The model under review builds one solid part; all positions refer to its coordinate system, in mm. A direction names the side the tool comes from. Give positions to 0.01 mm unless a question says otherwise; leave off trailing zeros. Loops run counter-clockwise (first coordinate to the right, second up) from the corner with the lowest first, then second, coordinate; pieces in that order, holes last. Notation, with made-up numbers: M 70.25,-20 L 115.25,-20 A28 cw 115.25,2 Z; hole C 68.5,88 d9. An arc over 180 degrees is marked long. Write item = value, one per line. Start each with the question number.
1. We need section C-C on x = 0. Give the boundary of the cut face in (y, z), then the cut area to 3 significant figures.
2. We need section D-D on z = 0. Count the separate pieces of the cut face and the enclosed holes in it, then the cut area to 3 significant figures.
3. We need section A-A on y = 17. Give the boundary of the cut face in (x, z), then the cut area to 3 significant figures.
4. Draft analysis for pull direction Y (two halves, no side actions). For faces 4 (the face through (-14.407, 42.605, 23.513)), 5 (the face through (-0.33, 29.53, -11.49)), 6 (the face through (11.51, 14.51, 0.55)), state which applies: pulls with the +Y half, pulls with the -Y half, needs draft (parallel to the pull), parting line crosses it, or undercut.
5. For pin 1 (1.5 mm diameter, centred on x = -6, z = -8.5, fed in from +Y); pin 2 (12.5 mm diameter, centred on x = 0.5, y = 22.5, fed in from -Z); pin 3 (4 mm diameter, centred on x = -9.5, z = -11, fed in from -Y); pin 4 (2 mm diameter, centred on x = -7.5, z = 16.5, fed in from -Y), all flat-tipped, find the tip position at first contact; note any pin that passes through.
6. Wall thickness on line 1 along Y through (x, z) = (11, 0); line 2 along X through (y, z) = (35.5, -24); line 3 along Z through (x, y) = (14.95, 36): over which ranges is each line inside the solid? List them lowest first. Write a range as from..to.
7. For faces 1 (the face through (12, 44, -25)), 2 (the face through (-10.5, 14, 0)), 3 (the face through (12.5, 17, 3)), list the 3-axis set-ups (+Z, -Z, +X, -X, +Y, -Y) from which the entire face can be reached by the end or side of a thin tool; tool diameter is ignored.
8. We need section B-B on y = 22.5. Give the boundary of the cut face in (x, z), then the cut area to 3 significant figures.
Autodesk Inventor part; units mm, degrees
ref_plane "YZ Plane" through (0, 0, 0) normal (1, 0, 0) x (0, 1, 0)
ref_plane "XZ Plane" through (0, 0, 0) normal (0, 1, 0) x (-1, 0, 0)
ref_plane "XY Plane" through (0, 0, 0) normal (0, 0, 1) x (1, 0, 0)
sketch "草圖1" plane through (0, 0, 0) normal (0, 1, 0) x (-1, 0, 0)
  line L0 (12.5, 12.5) -> (-12.5, 12.5)
  line L1 (-12.5, 12.5) -> (-12.5, -12.5)
  line L2 (-12.5, -12.5) -> (12.5, -12.5)
  line L3 (12.5, -12.5) -> (12.5, 12.5)
  line L4 (12.5, 12.5) -> (-12.5, -12.5) construction
  line L5 (-12.5, 12.5) -> (12.5, -12.5) construction
  point P0 (0, 0)
  dimension "d0" = 25
  dimension "d1" = 25
extrude "擠出1" add sketch "草圖1" along normal blind 35
sketch "草圖2" plane through (0, 35, 0) normal (0, 1, 0) x (1, 0, 0)
  line L0 (-10.5, -10.5) -> (10.5, -10.5)
  line L1 (10.5, -10.5) -> (10.5, 10.5)
  line L2 (10.5, 10.5) -> (-10.5, 10.5)
  line L3 (-10.5, 10.5) -> (-10.5, -10.5)
  line L4 (-10.5, -10.5) -> (10.5, 10.5) construction
  line L5 (10.5, -10.5) -> (-10.5, 10.5) construction
  point P0 (0, 0)
  dimension "d4" = 21
  dimension "d5" = 21
extrude "擠出2" cut sketch "草圖2" against normal through all
sketch "草圖3" plane through (-12.5, 0, 12.5) normal (0, 0, 1) x (1, 0, 0)
  line L0 (2, 35) -> (23, 35)
  line L1 (12.5, 35) -> (12.5, 0)
  circle A0 centre (12.5, 17) radius 2.55
  circle A1 centre (12.5, 27) radius 2.55
  line L2 (0, 0) -> (25, 0)
  point P0 (12.5, 0)
  dimension "d8" = 5.1
  dimension "d9" = 5.1
  dimension "d10" = 10
  dimension "d11" = 17
extrude "擠出3" cut sketch "草圖3" against normal through all
sketch "草圖4" plane through (0, 35, 0) normal (0, 1, 0) x (1, 0, 0)
  line L0 (-17.5, 27.5) -> (17.5, 27.5)
  line L1 (17.5, 27.5) -> (17.5, -27.5)
  line L2 (17.5, -27.5) -> (-17.5, -27.5)
  line L3 (-17.5, -27.5) -> (-17.5, 27.5)
  line L4 (-17.5, 27.5) -> (17.5, -27.5) construction
  line L5 (17.5, 27.5) -> (-17.5, -27.5) construction
  point P0 (0, 0)
  dimension "d14" = 55
  dimension "d15" = 35
extrude "擠出4" add sketch "草圖4" along normal blind 15
sketch "草圖5" plane through (0, 50, 0) normal (0, 1, 0) x (1, 0, 0)
  line L0 (-16, -22.5) -> (16, -22.5)
  line L1 (16, -22.5) -> (16, 22.5)
  line L2 (16, 22.5) -> (-16, 22.5)
  line L3 (-16, 22.5) -> (-16, -22.5)
  line L4 (-16, -22.5) -> (16, 22.5) construction
  line L5 (16, -22.5) -> (-16, 22.5) construction
  point P0 (0, 0)
  dimension "d18" = 45
  dimension "d19" = 32
extrude "擠出5" cut sketch "草圖5" against normal blind 12
sketch "草圖6" plane through (-17.5, 35, 27.5) normal (0, 0, 1) x (1, 0, 0)
  line L0 (0, 0) -> (0, 15)
  line L1 (0, 7.5) -> (35, 7.5)
  line L2 (35, 0) -> (35, 15)
  arc A0 (5.5, 7.5) -> (14.5, 7.5) centre (10, 7.5) ccw
  arc A1 (20.5, 7.5) -> (29.5, 7.5) centre (25, 7.5) ccw
  line L3 (35, 15) -> (0, 15)
  line L4 (17.5, 15) -> (17.5, 0)
  line L5 (0, 0) -> (35, 0)
  line L6 (5.5, 7.5) -> (14.5, 7.5)
  line L7 (14.5, 7.5) -> (14.5, 15)
  line L8 (14.5, 15) -> (5.5, 15)
  line L9 (5.5, 15) -> (5.5, 7.5)
  line L10 (20.5, 7.5) -> (29.5, 7.5)
  line L11 (29.5, 7.5) -> (29.5, 15)
  line L12 (29.5, 15) -> (20.5, 15)
  line L13 (20.5, 15) -> (20.5, 7.5)
  line L14 (14.5, 7.5) -> (20.5, 7.5)
  line L15 (1.5, 3) -> (33.5, 3)
  line L16 (5.5, 15) -> (29.5, 15)
  line L17 (29.5, 15) -> (29.5, 3)
  line L18 (29.5, 3) -> (5.5, 3)
  line L19 (5.5, 3) -> (5.5, 15)
  point P0 (17.5, -35)
  point P1 (20.5, 15)
  point P2 (29.5, 7.5)
  point P3 (28.5, 7.5)
  point P4 (29.5, 7.5)
  point P5 (5.5, 15)
  point P6 (14.5, 7.5)
  point P7 (13.5, 7.5)
  point P8 (25, 3)
  point P9 (10, 3)
  point P10 (25, 3)
  point P11 (29.5, 7.5)
  point P12 (5.5, 7.5)
  point P13 (5.5, 7.5)
  point P14 (29.5, 7.5)
  dimension "d22" = 9
  dimension "d23" = 9
  dimension "d24" = 15
  dimension "d25" = 7.5
  dimension "d52" = 24
extrude "擠出8" cut sketch "草圖6" against normal through all contours L9 L3 L7 L1 | L1 A0 | A0 L15 L19 | L15 A0 L1 L4 | L4 L1 A1 L15 | L7 L3 L4 L1 | L4 L3 L13 L1 | A1 L1 | A1 L17 L15 | L13 L3 L11 L1
sketch "草圖9" plane through (0, 50, 0) normal (0, 1, 0) x (1, 0, 0)
  circle A0 centre (-14.2115, -25) radius 1.5
  circle A1 centre (14.6091, -25) radius 1.5
  circle A2 centre (14.6091, 25.0995) radius 1.5
  circle A3 centre (-14.75, 25.0995) radius 1.5
  line L0 (-12, -27.5) -> (-12, -22.5)
  line L1 (-12, -25) -> (-17.5, -25)
  line L2 (-17.5, 27.5) -> (-17.5, -27.5)
  line L3 (17.5, -27.5) -> (17.5, 27.5)
  line L4 (17.5, -25) -> (-17.5, -25)
  line L5 (-17.5, 25.0938) -> (17.5, 25.0938)
  line L6 (14.6091, -25) -> (14.6091, 25.0995)
  line L7 (17.5, 27.5) -> (12, 27.5)
  line L8 (14.6091, 25.0995) -> (-14.75, 25.0995)
  line L9 (-14.75, 25.0995) -> (-14.75, -25)
  point P0 (0, 0)
  dimension "d34" = 3
  dimension "d35" = 3
  dimension "d36" = 3
  dimension "d37" = 3
  dimension "d38" = 0
  dimension "d39" = 0
extrude "擠出9" cut sketch "草圖9" against normal blind 15 contours L1 L9 A0 | A0 L1 | L9 L1 A0 | L9 L5 A3 | A3 L5 L9 | L4 A1 | A1 L6 L4 | A3 L8 L9 L5 | L5 L9 L8 A3 | L8 L6 L5 | A2 L5 L6 L8 | L5 L6 A2 | A1 L4 L6 | L6 L5 A2
sketch "草圖11" plane through (12.5, 0, 12.5) normal (1, 0, 0) x (0, 0, -1)
  circle A0 centre (12.5, 27) radius 2.55
  circle A1 centre (12.5, 17) radius 2.55
  line L0 (0, 0) -> (25, 0)
  point P0 (12.5, 0)
  point P1 (12.5, 0)
  dimension "d46" = 5.1
  dimension "d47" = 5.1
  dimension "d48" = 17
  dimension "d49" = 10
extrude "擠出11" cut sketch "草圖11" against normal up to surface (25 mm away)
sketch "草圖12" plane through (0, 38, 0) normal (0, 1, 0) x (1, 0, 0)
  circle A0 centre (-14.95, 21.45) radius 1.05
  circle A1 centre (14.95, 21.45) radius 1.05
  line L0 (-16, 22.5) -> (-12, 22.5)
  line L1 (-16, -22.5) -> (-16, 22.5)
  line L2 (12, 22.5) -> (16, 22.5)
  line L3 (16, 22.5) -> (16, -22.5)
  circle A2 centre (-14.95, -16.55) radius 1.05
  circle A3 centre (14.95, -16.55) radius 1.05
  point P0 (0, 0)
  dimension "d53" = 2.1
  dimension "d54" = 2.1
  dimension "d55" = 2.1
  dimension "d56" = 2.1
  dimension "d57" = 38
  dimension "d58" = 38
extrude "擠出12" cut sketch "草圖12" against normal up to surface (3 mm away) contours A0 | A2 | A1 | A3
Final values:
q1.outline = M 0,-12.5 L 14.45,-12.5 L 14.45,-10.5 L 0,-10.5 Z; M 0,10.5 L 14.45,10.5 L 14.45,12.5 L 0,12.5 Z; M 19.55,-12.5 L 24.45,-12.5 L 24.45,-10.5 L 19.55,-10.5 Z; M 19.55,10.5 L 24.45,10.5 L 24.45,12.5 L 19.55,12.5 Z; M 29.55,-12.5 L 35,-12.5 L 35,-27.5 L 38,-27.5 L 38,27.5 L 35,27.5 L 35,12.5 L 29.55,12.5 L 29.55,10.5 L 35,10.5 L 35,-10.5 L 29.55,-10.5 Z
q1.area = 264 mm²
q2.separate_pieces = 5
q2.enclosed_holes = 0
q2.area = 240 mm²
q3.outline = M -12.5,-12.5 L -2.55,-12.5 L -2.55,-10.5 L -10.5,-10.5 L -10.5,-2.55 L -12.5,-2.55 Z; M -12.5,2.55 L -10.5,2.55 L -10.5,10.5 L -2.55,10.5 L -2.55,12.5 L -12.5,12.5 Z; M 2.55,-12.5 L 12.5,-12.5 L 12.5,-2.55 L 10.5,-2.55 L 10.5,-10.5 L 2.55,-10.5 Z; M 2.55,10.5 L 10.5,10.5 L 10.5,2.55 L 12.5,2.55 L 12.5,12.5 L 2.55,12.5 Z
q3.area = 143 mm²
q4.face_4 = needs draft
q4.face_5 = undercut
q4.face_6 = undercut
q5.pin_1 = 38
q5.pin_2 = -12.5
q5.pin_3 = 0
q5.pin_4 = 35
q6.line_1 = 0..14.45, 19.55..24.45, 29.55..38
q6.line_2 = -17.5..-15.77, -13.73..13.59, 15.63..17.5
q6.line_3 = -27.5..-26.56, -23.64..-22.5, -20.4..15.5, 17.6..23.54, 26.46..27.5
q7.face_1 = +Z, -Z, +Y
q7.face_2 = -Y
q7.face_3 = +Z, -Z, +X, -Y
q8.outline = M -12.5,-12.5 L 12.5,-12.5 L 12.5,12.5 L -12.5,12.5 Z; hole M -10.5,-10.5 L 10.5,-10.5 L 10.5,10.5 L -10.5,10.5 Z
q8.area = 184 mm²
